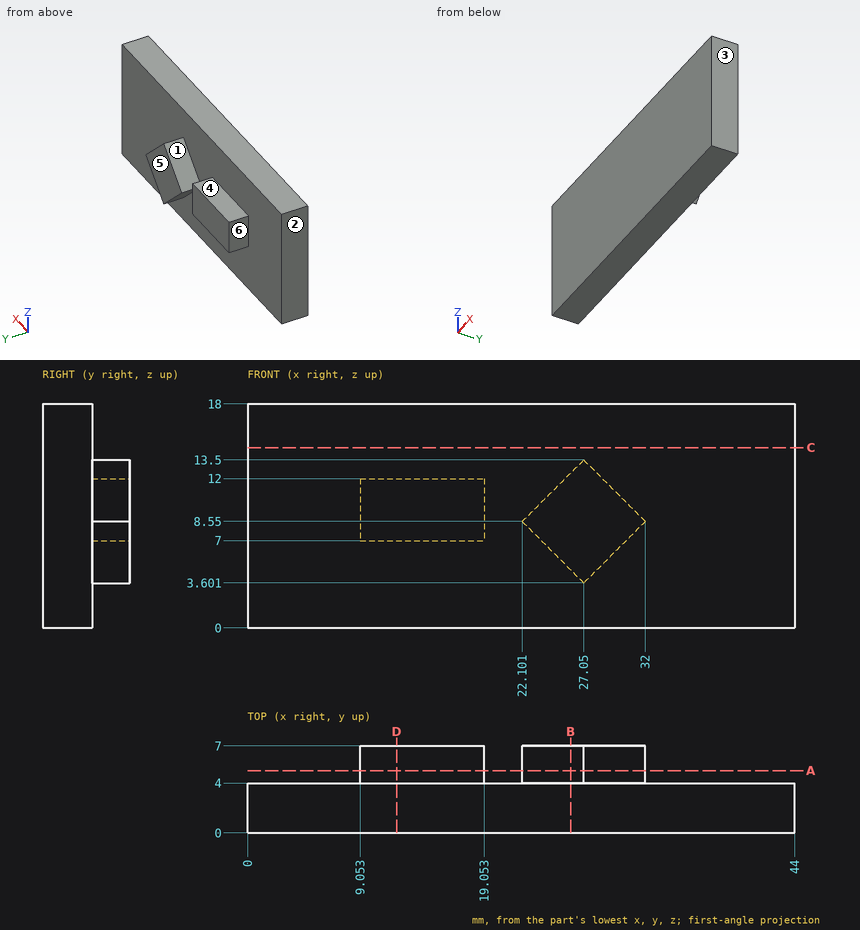
Print and shaded views of the part. All mm, measured from the part's lowest x, y and z. A direction names the side the tool comes from. Give positions to 0.01 mm unless a question says otherwise; leave off trailing zeros. Write each loop counter-clockwise with the first axis right and the second up, starting at its lowest first coordinate (ties: lowest second). Pieces come first, ordered by that corner, then holes. Notation, with made-up numbers: (39.5, -7) -> (59.5, -7) arc R23 cw to (59.5, 15) -> close; hole circle Ø6 at (84.25, 21). An arc over 180 degrees is marked (long way). Write item = value, one per line.
(1) Slice it at B-B, the plane x = 26. Give the cut face in (y, z).
Determined:
outline = (0, 0) -> (4, 0) -> (4, 4.65) -> (7, 4.65) -> (7, 12.45) -> (4, 12.45) -> (4, 18) -> (0, 18) -> close
(2) Slice it at C-C, the plane z = 14.5. Give the cut face in (x, y).
Determined:
outline = (0, 0) -> (44, 0) -> (44, 4) -> (0, 4) -> close
(3) Probe line 1 along Z through (x, y) = (19, 4.75); line 2 along Y through (x, z) = (22.5, 10.75); line 3 along X through (y, z) = (4.25, 5.75). List the from-to ranges inside material, lowest first.
Determined:
line_1 = 7 to 12
line_2 = 0 to 4
line_3 = 24.9 to 29.2
(4) Mould opens along X. For the marked faces 1, 2, 3 and 4 say: released by +X, released by -X, zero draft, split by the parting line, or undercut.
Determined:
face_1 = undercut
face_2 = released by -X
face_3 = released by +X
face_4 = zero draft
(5) Slice it at D-D, the plane x = 12. Give the cut face in (y, z), then the cut area to 3 significant figures.
Determined:
outline = (0, 0) -> (4, 0) -> (4, 7) -> (7, 7) -> (7, 12) -> (4, 12) -> (4, 18) -> (0, 18) -> close
area = 87.0 mm2
(6) Flat gauge pins, fed straight in: P1, Ø1.5, axis at y = 5, z = 10, coming from the +X side; P2, Ø2.5, axis at x = 13, y = 5.5, coming from the +Z side; P3, Ø0.9, axis at y = 5, z = 9, coming from the -X side. Where does each tip first touch, or does it go through?
Determined:
P1 = 31.3
P2 = 12
P3 = 9.05
(7) Slice it at A-A, the plane y = 5. Give the cut face in (x, z).
Determined:
outline = (9.05, 7) -> (19.05, 7) -> (19.05, 12) -> (9.05, 12) -> close; (22.1, 8.55) -> (27.05, 3.6) -> (32, 8.55) -> (27.05, 13.5) -> close
(8) Tool access for the marked faces 5 and 6: list every direction of +Z, -Z, +X, -X, +Y, -Y with a clear straight run to the whole face (end or side of a thin tool).
Determined:
face_5 = +Z, -Z, +X, -X, +Y
face_6 = +Z, -Z, -X, +Y
